Autodesk Inventor part; units mm, degrees
ref_plane "YZ Plane" through (0, 0, 0) normal (1, 0, 0) x (0, 1, 0)
ref_plane "XZ Plane" through (0, 0, 0) normal (0, 1, 0) x (-1, 0, 0)
ref_plane "XY Plane" through (0, 0, 0) normal (0, 0, 1) x (1, 0, 0)
sketch "Sketch1" plane through (0, 0, 0) normal (0, 1, 0) x (-1, 0, 0)
  line L0 (-105, 150) -> (105, 150)
  line L1 (105, 150) -> (105, -150)
  line L2 (105, -150) -> (-105, -150)
  line L3 (-105, -150) -> (-105, 150)
  line L4 (-105, 150) -> (105, -150) construction
  line L5 (105, 150) -> (-105, -150) construction
  circle A0 centre (-55, 130) radius 5
  circle A1 centre (55, 130) radius 5
  circle A2 centre (55, -100) radius 5
  circle A3 centre (-55, -100) radius 5
  point P0 (0, 0)
  dimension "d0" = 210
  dimension "d1" = 300
  dimension "d2" = 50
  dimension "d3" = 10
  dimension "d4" = 20
  dimension "d5" = 50
  dimension "d6" = 20
  dimension "d7" = 50
  dimension "d8" = 50
  dimension "d9" = 50
  dimension "d10" = 50
extrude "Extrusion1" add sketch "Sketch1" along normal blind 3
sketch "Sketch2" plane through (0, 0, 0) normal (0, -1, 0) x (1, 0, 0)
  circle A0 centre (-55, 130) radius 5
  circle A1 centre (-55, 130) radius 11
  circle A2 centre (55, 130) radius 5
  circle A3 centre (55, 130) radius 11
  point P0 (0, 0)
  dimension "d13" = 22
extrude "Extrusion2" cut sketch "Sketch2" against normal blind 1
ref_plane "Work Plane1" through (0, 0, 150) normal (1, 0, 0) x (0, 0, -1)
equation "\"d5\" = d2"
equation "\"d8\" = d2"
equation "\"d10\" = d2"
properties part number "chasis"
Part model, mm, in its own coordinate system. A direction names the side the tool comes from. Coordinates: 2 decimals unless noted, no trailing zeros. Write each loop counter-clockwise with the first axis right and the second up, starting at its lowest first coordinate (ties: lowest second). Pieces come first, ordered by that corner, then holes.
Item 1: Slice it at A-A (z = -100). Write the cut outline in (x, y).
Item 2: Probe line 1 (Z direction, x = 55, y = 2.4); line 2 (Z direction, x = 55, y = 0.5); line 3 (X direction, y = 1.7, z = 130). List the from-to ranges inside material, lowest first.
Item 3: Slice it at C-C (z = 130). Write the cut outline in (x, y), and give its area (3 significant figures).
Item 4: Slice it at B-B (x = -55). Write the cut outline in (y, z).
Item 5: Which spindle directions (+Z, -Z, +X, -X, +Y, -Y) get a long thin tool onto all of the face, cutting with end or side? Do faces 4 (the face through (59, 1, -103)), 5 (the face through (53.568, 0.493, 140.906)). Say none if no direction does.
Item 6: Pin check, flat tips, straight feed: pin 1 (12 mm diameter, centred on x = -38.5, z = 91, fed in from -Y); pin 2 (6 mm diameter, centred on x = -55, z = 130, fed in from +Y); pin 3 (16 mm diameter, centred on x = 55, z = 130, fed in from -Y). Stop position of each tip, or through.
Item 7: Mould opens along Z. For faces 1 (the face through (1, 0, 2)), 2 (the face through (-53, 1, 125)), 3 (the face through (-51, 1, -103)) say: released by +Z, released by -Z, zero draft, split by the parting line, or undercut.
Results found:
1. outline: (-105, 0) - (-60, 0) - (-60, 3) - (-105, 3) - close; (-50, 0) - (50, 0) - (50, 3) - (-50, 3) - close; (60, 0) - (105, 0) - (105, 3) - (60, 3) - close
2. line 1: z = -150 to -105, -95 to 125, 135 to 150
2. line 2: z = -150 to -105, -95 to 119, 141 to 150
2. line 3: x = -105 to -60, -50 to 50, 60 to 105
3. outline: (-105, 0) - (-66, 0) - (-66, 1) - (-60, 1) - (-60, 3) - (-105, 3) - close; (-50, 1) - (-44, 1) - (-44, 0) - (44, 0) - (44, 1) - (50, 1) - (50, 3) - (-50, 3) - close; (60, 1) - (66, 1) - (66, 0) - (105, 0) - (105, 3) - (60, 3) - close
3. area: 546 mm2
4. outline: (0, -150) - (3, -150) - (3, -105) - (0, -105) - close; (0, -95) - (3, -95) - (3, 125) - (1, 125) - (1, 119) - (0, 119) - close; (0, 141) - (1, 141) - (1, 135) - (3, 135) - (3, 150) - (0, 150) - close
5. face 4: +Y, -Y
5. face 5: -Y
6. pin 1: stops at y = 0
6. pin 2: passes through
6. pin 3: stops at y = 1
7. face 1: zero draft
7. face 2: undercut
7. face 3: undercut
